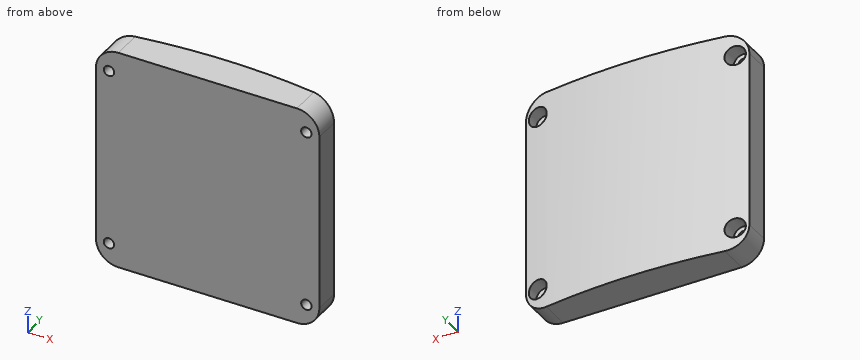
from build123d import *

# Parameters (mm, degrees)
BOSS_EXTRUDE1_DEPTH             = 31.623
FILLET1_R                       = 6.35
F_32_0_116_DIAMETER_HOLE1_D     = 2.9464
F_32_0_116_DIAMETER_HOLE1_DEPTH = 3.81
SKETCH7_R                       = 2.7813
CUT_EXTRUDE4_DEPTH              = 46.170242106


with BuildPart() as part:
    # Sketch1 → Boss-Extrude1 (new, symmetric)
    with BuildSketch(Plane.XY):
        with BuildLine():
            Line((-31.623, 174.965213317), (-31.623, 167.64))
            Line((-31.623, 167.64), (-24.003, 167.64))
            Line((-24.003, 167.64), (24.003, 167.64))
            Line((24.003, 167.64), (31.623, 167.64))
            Line((31.623, 167.64), (31.623, 174.965213317))
            ThreePointArc((31.623, 174.965213317), (0, 177.8), (-31.623, 174.965213317))
        make_face()
    extrude(amount=BOSS_EXTRUDE1_DEPTH, both=True)

    # Fillet1
    fillet1_edges = [part.edges().sort_by_distance(p)[0] for p in [
        (31.623, 171.302606658, 31.623),
        (31.623, 171.302606658, -31.623),
        (-31.623, 171.302606658, 31.623),
        (-31.623, 171.302606658, -31.623),
    ]]
    fillet(fillet1_edges, radius=FILLET1_R)

    # 32 _0.116_ Diameter Hole1
    with Locations(Plane.XZ.offset(-167.64)):
        with Locations((27.94, -25.4), (-27.94, -25.4), (27.94, 25.4), (-27.94, 25.4)):
            Hole(F_32_0_116_DIAMETER_HOLE1_D / 2, depth=F_32_0_116_DIAMETER_HOLE1_DEPTH)

    # Sketch7 → Cut-Extrude4 (cut, through all)
    with BuildSketch(Plane.XZ.offset(-171.45)):
        with Locations(Location((27.94, -25.4, 0), (0, 0, 270))):
            Circle(SKETCH7_R)
        with Locations(Location((27.94, 25.4, 0), (0, 0, 270))):
            Circle(SKETCH7_R)
        with Locations(Location((-27.94, 25.4, 0), (0, 0, 270))):
            Circle(SKETCH7_R)
        with Locations(Location((-27.94, -25.4, 0), (0, 0, 270))):
            Circle(SKETCH7_R)
    extrude(amount=-CUT_EXTRUDE4_DEPTH, mode=Mode.SUBTRACT)


solid = part.part
Part model, mm, in its own coordinate system. Round coordinates to 2 decimals unless told otherwise and drop trailing zeros. Write each loop counter-clockwise with the first axis right and the second up, starting at its lowest first coordinate (ties: lowest second). Pieces come first, ordered by that corner, then holes. Notation, with made-up numbers: M 8.5,-35.5 L 67.5,-35.5 A13 ccw 67.5,-12.5 Z; hole C -27.75,-32 d5. An arc over 180 degrees is marked long. Return JSON: item names as keys, results as strings. Group by question number.
(1) Saw through at C-C on z = -15.5. Write the cut outline in (x, y), then the cut area to 3 significant figures.
(2) Pin check, flat tips, straight feed: pin 1 Ø2.5 at (x, z) = (-27.94, 25.4) entering from +Y; pin 2 Ø6 at (x, z) = (29, 25.5) entering from +Y; pin 3 Ø4.5 at (x, z) = (27.94, 25.4) entering from +Y; pin 4 Ø9 at (x, z) = (-27.94, -25.4) entering from +Y. Stop position of each tip, or through.
(3) Saw through at D-D on x = -8.5. Write the cut outline in (y, z).
(4) Saw through at B-B on y = 172.75. Write the cut outline in (x, z), then the cut area to 3 significant figures.
(5) Saw through at A-A on x = -27.94. Write the cut outline in (y, z).
(6) Drill centre lines: probe 1 along X at (y, z) = (172.7, 25.4); probe 2 along Z at (x, y) = (-28.5, 175); probe 3 along Z at (x, y) = (-28, 170.75). Where is each one in solid material? Low to high.
Returned:
{
 "1": {"outline": "M -31.62,167.64 L 31.62,167.64 L 31.62,174.97 A177.8 ccw -31.62,174.97 Z", "area": "583 mm²"},
 "2": {"pin 1": "through", "pin 2": "y = 175.64", "pin 3": "y = 171.45", "pin 4": "y = 176.25"},
 "3": {"outline": "M 167.64,-31.62 L 177.6,-31.62 L 177.6,31.62 L 167.64,31.62 Z"},
 "4": {"outline": "M -31.62,-25.27 A6.35 ccw -25.27,-31.62 L 25.27,-31.62 A6.35 ccw 31.62,-25.27 L 31.62,25.27 A6.35 ccw 25.27,31.62 L -25.27,31.62 A6.35 ccw -31.62,25.27 Z; hole C -27.94,-25.4 d5.56; hole C -27.94,25.4 d5.56; hole C 27.94,-25.4 d5.56; hole C 27.94,25.4 d5.56", "area": "3,870 mm²"},
 "5": {"outline": "M 167.64,-31.04 L 175.59,-31.04 L 175.59,-28.18 L 171.45,-28.18 L 171.45,-26.87 L 167.64,-26.87 Z; M 167.64,-23.93 L 171.45,-23.93 L 171.45,-22.62 L 175.59,-22.62 L 175.59,22.62 L 171.45,22.62 L 171.45,23.93 L 167.64,23.93 Z; M 167.64,26.87 L 171.45,26.87 L 171.45,28.18 L 175.59,28.18 L 175.59,31.04 L 167.64,31.04 Z"},
 "6": {"probe 1": "-31.62 to -30.72, -25.16 to 25.16, 30.72 to 31.62", "probe 2": "-30.74 to -28.12, -22.68 to 22.68, 28.12 to 30.74", "probe 3": "-31.01 to -26.87, -23.93 to 23.93, 26.87 to 31.01"}
}
